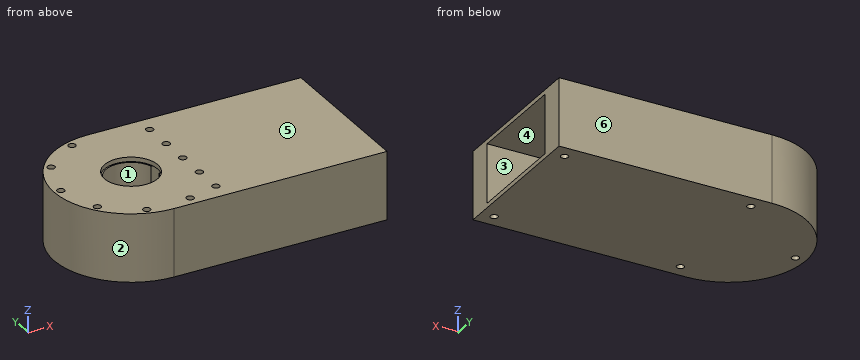
from build123d import *

# Parameters (mm, degrees)
SALIENTE_EXTRUIR1_DEPTH = 40
CROQUIS4_R              = 18
SALIENTE_EXTRUIR2_DEPTH = 3
SALIENTE_EXTRUIR3_START = 3
SALIENTE_EXTRUIR3_DEPTH = 3
CROQUIS6_R              = 2.5
CORTAR_EXTRUIR1_DEPTH   = 10
CROQUIS7_R              = 2.5
CORTAR_EXTRUIR2_DEPTH   = 25


with BuildPart() as part:
    # Croquis2 → Saliente-Extruir1 (new body)
    with BuildSketch(Plane.XY):
        with BuildLine():
            Line((144, 52), (0, 52))
            ThreePointArc((0, 52), (-52, 0), (0, -52))
            Line((0, -52), (144, -52))
            Line((144, -52), (144, -35))
            Line((144, -35), (40, -35))
            Line((40, -35), (40, -5))
            Line((40, -5), (16.248076809, -5))
            ThreePointArc((16.248076809, -5), (-17, 0), (16.248076809, 5))
            Line((16.248076809, 5), (40, 5))
            Line((40, 5), (40, 35))
            Line((40, 35), (144, 35))
            Line((144, 35), (144, 52))
        make_face()
    extrude(amount=SALIENTE_EXTRUIR1_DEPTH)

    # Croquis4 → Saliente-Extruir2 (add)
    with BuildSketch(Plane.XY.offset(40)):
        with BuildLine():
            Line((144, 52), (144, -52))
            Line((144, -52), (0, -52))
            ThreePointArc((0, -52), (-52, 0), (0, 52))
            Line((0, 52), (144, 52))
        make_face()
        with Locations(Location((0, 0, 0), (0, 0, 16.127620213))):
            Circle(CROQUIS4_R, mode=Mode.SUBTRACT)
    extrude(amount=SALIENTE_EXTRUIR2_DEPTH)

    # Croquis5 → Saliente-Extruir3 (add)
    with BuildSketch(Plane(origin=(0, 0, 0), x_dir=(-1, 0, 0), z_dir=(0, 0, -1)).offset(SALIENTE_EXTRUIR3_START)):
        with BuildLine():
            Line((0, -52), (-144, -52))
            Line((-144, -52), (-144, 52))
            Line((-144, 52), (0, 52))
            ThreePointArc((0, 52), (52, 0), (0, -52))
        make_face()
    extrude(amount=-SALIENTE_EXTRUIR3_DEPTH)

    # Croquis6 → Cortar-Extruir1 (cut)
    with BuildSketch(Plane(origin=(0, 0, -3), x_dir=(-1, 0, 0), z_dir=(0, 0, -1))):
        with Locations((-135, 42.5)):
            Circle(CROQUIS6_R)
        with Locations(Location((-9, 42.5, 0), (0, 0, 180))):
            Circle(CROQUIS6_R)
        with Locations((-9, -42.5)):
            Circle(CROQUIS6_R)
        with Locations(Location((-135, -42.5, 0), (0, 0, 180))):
            Circle(CROQUIS6_R)
        with Locations((45, 0)):
            Circle(CROQUIS6_R)
    extrude(amount=-CORTAR_EXTRUIR1_DEPTH, mode=Mode.SUBTRACT)

    # Croquis7 → Cortar-Extruir2 (cut)
    with BuildSketch(Plane.XY.offset(43)):
        with Locations((35, 0)):
            Circle(CROQUIS7_R)
        with Locations((35, 20)):
            Circle(CROQUIS7_R)
        with Locations((35, 40)):
            Circle(CROQUIS7_R)
        with Locations(Location((35, -40, 0), (0, 0, 180))):
            Circle(CROQUIS7_R)
        with Locations(Location((35, -20, 0), (0, 0, 180))):
            Circle(CROQUIS7_R)
        with Locations((-14.678307233, 45.175184524)):
            Circle(CROQUIS7_R)
        with Locations((-38.428307233, 27.919799484)):
            Circle(CROQUIS7_R)
        with Locations((-47.5, 0)):
            Circle(CROQUIS7_R)
        with Locations((-38.428307233, -27.919799484)):
            Circle(CROQUIS7_R)
        with Locations((-14.678307233, -45.175184524)):
            Circle(CROQUIS7_R)
        with Locations((14.678307233, -45.175184524)):
            Circle(CROQUIS7_R)
    extrude(amount=-CORTAR_EXTRUIR2_DEPTH, mode=Mode.SUBTRACT)


solid = part.part
CAD build for the part. Positions are in the model's coordinates, mm. Face numbers are marked on the shaded views. A direction names the side the tool comes from. Give positions to 0.01 mm unless a question says otherwise; leave off trailing zeros. Order: outer loops, then holes, each group sorted by start corner. A loop starts at its lowest first (then second) coordinate and runs counter-clockwise, first axis right, second up. Notation, with made-up numbers: (-22.5, 35) -> (11.5, 35) arc R29 cw to (11.5, 61) -> close; hole circle Ø1 at (27.5, -6.75). An arc over 180 degrees is marked (long way). Return JSON: item names as keys, results as strings.
Q1. Mould opens along Y. For the marked faces 4, 5 and 6 say: pulls with the +Y half, pulls with the -Y half, needs draft (parallel to the pull), parting line crosses it, or undercut.
Working result:
{"face 4": "undercut", "face 5": "needs draft", "face 6": "pulls with the +Y half"}
Q2. Drill centre lines: line 1 (Z direction, x = 61, y = -32.5); line 2 (Y direction, x = 41, z = 29.5); line 3 (Y direction, x = 0, z = 41.2). Where is each one in solid material? Low to high.
Working result:
{"line 1": "-3 to 0, 40 to 43", "line 2": "-52 to -35, 35 to 52", "line 3": "-52 to -18, 18 to 52"}
Q3. Saw through at A-A (y = 0). Write the cut outline in (x, z), then the cut area to 3 significant figures.
Working result:
{"outline": "(-52, -3) -> (-47.5, -3) -> (-47.5, 7) -> (-42.5, 7) -> (-42.5, -3) -> (144, -3) -> (144, 0) -> (-17, 0) -> (-17, 40) -> (-18, 40) -> (-18, 43) -> (-45, 43) -> (-45, 18) -> (-50, 18) -> (-50, 43) -> (-52, 43) -> close; (18, 40) -> (32.5, 40) -> (32.5, 43) -> (18, 43) -> close; (37.5, 40) -> (144, 40) -> (144, 43) -> (37.5, 43) -> close", "area": "2,280 mm²"}
Q4. Which spindle directions (+Z, -Z, +X, -X, +Y, -Y) get a long thin tool onto all of the face, cutting with end or side? Do the marked faces 1, 2 and 3. Say none if no direction does.
Working result:
{"face 1": "+Z", "face 2": "+Z, -Z, -X", "face 3": "+X"}
Q5. Saw through at D-D (y = -20). Write the cut outline in (x, z).
Working result:
{"outline": "(-48, -3) -> (144, -3) -> (144, 0) -> (40, 0) -> (40, 40) -> (144, 40) -> (144, 43) -> (37.5, 43) -> (37.5, 18) -> (32.5, 18) -> (32.5, 43) -> (-48, 43) -> close"}
Q6. Saw through at B-B (x = 74). Write the cut outline in (y, z).
Working result:
{"outline": "(-52, -3) -> (52, -3) -> (52, 43) -> (-52, 43) -> close; hole (-35, 0) -> (35, 0) -> (35, 40) -> (-35, 40) -> close"}
Q7. Saw through at C-C (z = 28). Count the separate pieces of the cut face and the enclosed holes in it, then the cut area to 3 significant figures.
Working result:
{"separate pieces": "1", "enclosed holes": "10", "area": "10,600 mm²"}
Q8. Flat gauge pins, fed straight in: pin 1 (4.5 mm diameter, centred on x = 35, y = 40, fed in from +Z); pin 2 (4 mm diameter, centred on y = -19.5, z = 2.5, fed in from +X); pin 3 (2.5 mm diameter, centred on x = 10, y = -42, fed in from -Z). Where does each tip first touch, or does it go through?
Working result:
{"pin 1": "z = 18", "pin 2": "x = 40", "pin 3": "z = 7"}
